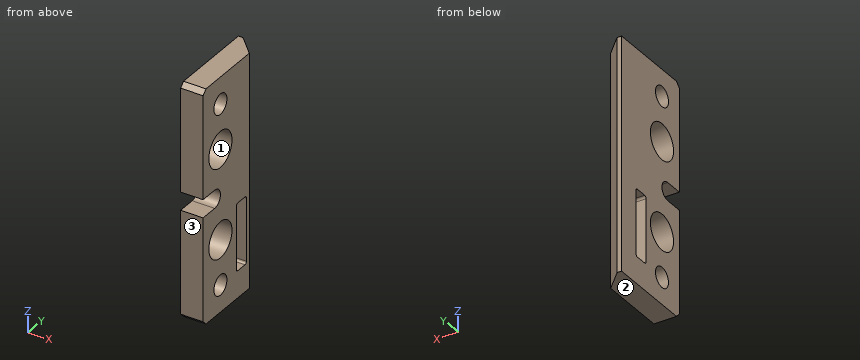
from build123d import *

# Parameters (mm, degrees)
SKETCH1_W           = 5
SKETCH1_H           = 20
BOSS_EXTRUDE1_DEPTH = 52
SKETCH2_R           = 2.25
SKETCH2_R_2         = 4
SKETCH2_W           = 15
SKETCH2_H           = 3.5
CUT_EXTRUDE1_DEPTH  = 52
FILLET1_R           = 0.5
CHAMFER1_SIZE       = 1
CHAMFER2_SIZE       = 4


with BuildPart() as part:
    # Sketch1 → Boss-Extrude1 (new body)
    with BuildSketch(Plane.XY):
        with Locations((1.671974522, -6.576433121)):
            Rectangle(SKETCH1_W, SKETCH1_H)
    extrude(amount=BOSS_EXTRUDE1_DEPTH)

    # Sketch2 → Cut-Extrude1 (cut)
    with BuildSketch(Plane(origin=(4.171974522, 0, 0), x_dir=(0, 0, -1), z_dir=(1, 0, 0))):
        with Locations((-46, -10.576433121)):
            Circle(SKETCH2_R)
        with Locations((-36, -10.576433121)):
            Circle(SKETCH2_R_2)
        with Locations((-16, -10.576433121)):
            Circle(SKETCH2_R_2)
        with Locations((-6, -10.576433121)):
            Circle(SKETCH2_R)
        with BuildLine():
            Line((-23.99, -16.576433121), (-28.01, -16.576433121))
            Line((-28.01, -16.576433121), (-28.01, -12.576433121))
            ThreePointArc((-28.01, -12.576433121), (-26, -10.566433121), (-23.99, -12.576433121))
            Line((-23.99, -12.576433121), (-23.99, -16.576433121))
        make_face()
        with Locations((-13.5, -3.326433121)):
            Rectangle(SKETCH2_W, SKETCH2_H)
    extrude(amount=-CUT_EXTRUDE1_DEPTH, mode=Mode.SUBTRACT)

    # Fillet1
    fillet1_edges = [part.edges().sort_by_distance(p)[0] for p in [
        (1.671974522, -5.076433121, 21),
        (1.671974522, -1.576433121, 21),
        (1.671974522, -1.576433121, 6),
        (1.671974522, -5.076433121, 6),
    ]]
    fillet(fillet1_edges, radius=FILLET1_R)

    # Chamfer1
    chamfer1_edges = [part.edges().sort_by_distance(p)[0] for p in [
        (1.671974522, -16.576433121, 0),
        (1.671974522, -16.576433121, 52),
    ]]
    chamfer(chamfer1_edges, length=CHAMFER1_SIZE)

    # Chamfer2
    chamfer2_edges = [part.edges().sort_by_distance(p)[0] for p in [
        (4.171974522, 3.423566879, 26),
    ]]
    chamfer(chamfer2_edges, length=CHAMFER2_SIZE)


solid = part.part
Input: part model. Units: mm. Frame: model coordinates. Face numbers are marked on the shaded views. Give positions to 0.01 mm unless a question says otherwise; leave off trailing zeros. Loops run counter-clockwise (first coordinate to the right, second up) from the corner with the lowest first, then second, coordinate; pieces in that order, holes last. Notation, with made-up numbers: M 72,32 L 87,32 A5 cw 87,36 Z; hole C 33,62 d4. An arc over 180 degrees is marked long. Use CSV: the item, a comma, the result in double quotes.
(1) Material intervals for L1, parallel to Z at x = 0.4, y = -13.25; L2, parallel to Z at x = 1.95, y = -12.5; L3, parallel to Z at x = 2.05, y = -2, sorted ascending. Write a range as [from, to].
Outcome:
L1,"z = [0, 13.02], [18.98, 23.99], [28.01, 33.02], [38.98, 52]"
L2,"z = [0, 4.83], [7.17, 12.49], [19.51, 23.99], [28.01, 32.49], [39.51, 44.83], [47.17, 52]"
L3,"z = [0, 6.01], [20.99, 52]"
(2) Section D-D, the plane x = 3.3. Return loops of the section in (y, z).
Outcome:
outline,"M -16.58,1 L -15.58,0 L 0.3,0 L 0.3,52 L -15.58,52 L -16.58,51 L -16.58,28.01 L -12.58,28.01 A2.01 cw -12.58,23.99 L -16.58,23.99 Z; hole C -10.58,16 d8; hole C -10.58,36 d8; hole C -10.58,6 d4.5; hole C -10.58,46 d4.5; hole M -5.08,6.5 A0.5 ccw -4.58,6 L -2.08,6 A0.5 ccw -1.58,6.5 L -1.58,20.5 A0.5 ccw -2.08,21 L -4.58,21 A0.5 ccw -5.08,20.5 Z"
(3) Pull-direction query (Y, two-part tool) for the marked faces 1, 2 and 3; classes: pulls with the +Y half, pulls with the -Y half, needs draft (parallel to the pull), parting line crosses it, or undercut.
Outcome:
face 1,"undercut"
face 2,"needs draft"
face 3,"pulls with the -Y half"
(4) Section C-C, the plane z = 36. Return loops of the section in (x, y).
Outcome:
outline,"M -0.83,-16.58 L 4.17,-16.58 L 4.17,-14.58 L -0.83,-14.58 Z; M -0.83,-6.58 L 4.17,-6.58 L 4.17,-0.58 L 0.17,3.42 L -0.83,3.42 Z"
(5) Section B-B, the plane y = -9. Return loops of the section in (x, z), plus the area to 3 significant figures.
Outcome:
outline,"M -0.83,0 L 4.17,0 L 4.17,4.39 L -0.83,4.39 Z; M -0.83,7.61 L 4.17,7.61 L 4.17,12.32 L -0.83,12.32 Z; M -0.83,19.68 L 4.17,19.68 L 4.17,32.32 L -0.83,32.32 Z; M -0.83,39.68 L 4.17,39.68 L 4.17,44.39 L -0.83,44.39 Z; M -0.83,47.61 L 4.17,47.61 L 4.17,52 L -0.83,52 Z"
area,"154 mm²"
(6) Section A-A, the plane z = 16. Return loops of the section in (x, y), plus the area to 3 significant figures.
Outcome:
outline,"M -0.83,-16.58 L 4.17,-16.58 L 4.17,-14.58 L -0.83,-14.58 Z; M -0.83,-6.58 L 4.17,-6.58 L 4.17,-5.08 L -0.83,-5.08 Z; M -0.83,-1.58 L 4.17,-1.58 L 4.17,-0.58 L 0.17,3.42 L -0.83,3.42 Z"
area,"34.5 mm²"
(7) Pin query (flat end, axial travel): P1, Ø7, axis at y = -10.58, z = 16, coming from the +X side. Return the tip coordinate at first contact, or that it passes through.
Outcome:
P1,"passes through"
